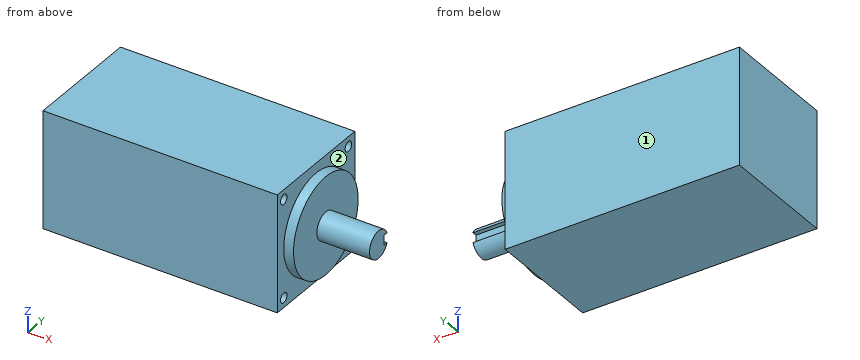
from build123d import *

# Parameters (mm, degrees)
SKETCH_1_W          = 60
SKETCH_1_H          = 60
EXTRUDE_1_DEPTH     = 120
SKETCH_2_R          = 2.5
CUT_EXTRUDE_1_DEPTH = 20
SKETCH_3_R          = 25
EXTRUDE_2_DEPTH     = 5
SKETCH_4_R          = 7
EXTRUDE_3_DEPTH     = 27
SKETCH_5_W          = 5
SKETCH_5_H          = 2.748835856
CUT_EXTRUDE_2_DEPTH = 27


with BuildPart() as part:
    # 草图1 → 凸台-拉伸1 (new body)
    with BuildSketch(Plane(origin=(0, 0, 0), x_dir=(0, 0, -1), z_dir=(1, 0, 0))):
        Rectangle(SKETCH_1_W, SKETCH_1_H)
    extrude(amount=-EXTRUDE_1_DEPTH)

    # 草图2 → 切除-拉伸1 (cut)
    with BuildSketch(Plane(origin=(0, 0, 0), x_dir=(0, 0, -1), z_dir=(1, 0, 0))):
        with Locations((-25, 25)):
            Circle(SKETCH_2_R)
        with Locations((25, 25)):
            Circle(SKETCH_2_R)
        with Locations((-25, -25)):
            Circle(SKETCH_2_R)
        with Locations((25, -25)):
            Circle(SKETCH_2_R)
    extrude(amount=-CUT_EXTRUDE_1_DEPTH, mode=Mode.SUBTRACT)

    # 草图3 → 凸台-拉伸2 (add)
    with BuildSketch(Plane(origin=(0, 0, 0), x_dir=(0, 0, -1), z_dir=(1, 0, 0))):
        Circle(SKETCH_3_R)
    extrude(amount=EXTRUDE_2_DEPTH)

    # 草图4 → 凸台-拉伸3 (add)
    with BuildSketch(Plane(origin=(5, 0, 0), x_dir=(0, 0, -1), z_dir=(1, 0, 0))):
        Circle(SKETCH_4_R)
    extrude(amount=EXTRUDE_3_DEPTH)

    # 草图5 → 切除-拉伸2 (cut)
    with BuildSketch(Plane(origin=(32, 0, 0), x_dir=(0, 0, -1), z_dir=(1, 0, 0))):
        with Locations((0, 5.625582072)):
            Rectangle(SKETCH_5_W, SKETCH_5_H)
    extrude(amount=-CUT_EXTRUDE_2_DEPTH, mode=Mode.SUBTRACT)


solid = part.part
Read the model definition and answer for the solid it produces. Units are mm, in the model's axes. Face numbers are marked on the shaded views. A direction names the side the tool comes from. Round coordinates to 2 decimals unless told otherwise and drop trailing zeros. Write each loop counter-clockwise with the first axis right and the second up, starting at its lowest first coordinate (ties: lowest second). Pieces come first, ordered by that corner, then holes.
Q1. Find section A-A on z = 0. Determine the outline of the cut face in (x, y).
Values:
outline: (-120, -30) - (0, -30) - (0, -25) - (5, -25) - (5, -7) - (32, -7) - (32, 4.25) - (5, 4.25) - (5, 25) - (0, 25) - (0, 30) - (-120, 30) - close
Q2. Find section B-B on y = 0. Determine the outline of the cut face in (x, z).
Values:
outline: (-120, -30) - (0, -30) - (0, -25) - (5, -25) - (5, -7) - (32, -7) - (32, 7) - (5, 7) - (5, 25) - (0, 25) - (0, 30) - (-120, 30) - close
Q3. A tool of negligible diameter and unlimited length cuts with its end or side. For the marked faces 1 and 2, from which of +Z, -Z, +X, -X, +Y, -Y can it reach the whole face along a straight path? Write none if from no direction.
Values:
face 1: +Z, -Z, +X, -X, +Y
face 2: +X
Q4. Find section C-C on z = 14. Determine the outline of the cut face in (x, y).
Values:
outline: (-120, -30) - (0, -30) - (0, -20.71) - (5, -20.71) - (5, 20.71) - (0, 20.71) - (0, 30) - (-120, 30) - close
Q5. Flat-ended cylindrical pins translate along their axes: P1, Ø2.5, axis at y = -25, z = -25, coming from the +X side; P2, Ø8, axis at y = -14, z = 13, coming from the +X side; P3, Ø5.5, axis at y = 26, z = -25.5, coming from the +X side. Find the tip coordinate at first contact, or state that the pin passes through.
Values:
P1: stops at x = -20
P2: stops at x = 5
P3: stops at x = 0
Q6. Straight lines are drawn through the part: line 1 (X direction, y = 9, z = 26.5); line 2 (X direction, y = -3, z = -12.5); line 3 (Y direction, x = 19, z = 4). For each, find the intervals that lie inside material, in ascending order.
Values:
line 1: x = -120 to 0
line 2: x = -120 to 5
line 3: y = -5.74 to 5.74
